Model file for the job. Use its own axes, mm. A direction names the side the tool comes from. Coordinates: 2 decimals unless noted, no trailing zeros. Order: outer loops, then holes, each group sorted by start corner. A loop starts at its lowest first (then second) coordinate and runs counter-clockwise, first axis right, second up. Notation, with made-up numbers: M 68,-3 L 122,-3 A11 cw 122,16 Z; hole C -8,84.25 d2. An arc over 180 degrees is marked long. Return JSON: item names as keys, results as strings.
```python
from build123d import *

# Parameters (mm, degrees)
F0_W     = 76.5
F0_H     = 16.5
F2_DEPTH = 2
F1_R     = 2.25
F3_DEPTH = 1
F4_R     = 2


with BuildPart() as f2:
    # F0 (on Front) → F2 (new body)
    with BuildSketch(Plane.XZ):
        Rectangle(F0_W, F0_H)
    extrude(amount=-F2_DEPTH)

    # F1 (on Front) → F3 (join)
    with BuildSketch(Plane.XZ):
        with Locations((-35.5, 5.8)):
            Circle(F1_R)
        with Locations((35.5, -5.8)):
            Circle(F1_R)
    extrude(amount=F3_DEPTH)

    # F4
    f4_edges = [f2.edges().sort_by_distance(p)[0] for p in [
        (38.25, 1, -8.25),
        (38.25, 1, 8.25),
        (-38.25, 1, -8.25),
        (-38.25, 1, 8.25),
    ]]
    fillet(f4_edges, radius=F4_R)


solid = f2.part
```
Item 1: Saw through at A-A (x = -35.5). Write the cut outline in (y, z).
Check result:
{"outline": "M -1,3.55 L 0,3.55 L 0,-8.25 L 2,-8.25 L 2,8.25 L 0,8.25 L 0,8.05 L -1,8.05 Z"}
Item 2: 3-axis set-ups, long thin cutter, end or side, ignore diameter. For faces 1 (the cylindrical face through (-33.42, -0.49, 4.94)), 2 (the cylindrical face through (37.65, 1.01, -7.68)): which of +Z, -Z, +X, -X, +Y, -Y reach the whole face in a straight line?
Check result:
{"face 1": "-Y", "face 2": "-Z, +X, +Y, -Y"}
Item 3: Saw through at B-B (z = 1). Write the cut outline in (x, y), and give its area (3 significant figures).
Check result:
{"outline": "M -38.25,0 L 38.25,0 L 38.25,2 L -38.25,2 Z", "area": "153 mm2"}
Item 4: Saw through at C-C (x = 24). Write the cut outline in (y, z).
Check result:
{"outline": "M 0,-8.25 L 2,-8.25 L 2,8.25 L 0,8.25 Z"}
Item 5: Wall check: line 1 (Y direction, x = -17, z = 3.5); line 2 (X direction, y = -0.6, z = -5.75); line 3 (X direction, y = -0.8, z = 6.5). Give the ranges that are in metal, low to high.
Check result:
{"line 1": "y = 0 to 2", "line 2": "x = 33.25 to 37.75", "line 3": "x = -37.64 to -33.36"}
